CAD build for the part. Positions are in the model's coordinates, mm. Give positions to 0.01 mm unless a question says otherwise; leave off trailing zeros. Loops run counter-clockwise (first coordinate to the right, second up) from the corner with the lowest first, then second, coordinate; pieces in that order, holes last.
Item 1: Saw through at A-A on x = 0. Give the cut face in (y, z), plus the area to 3 significant figures.
Item 2: Drop flat-ended pins along their axis: P1, Ø22.5, axis at x = 171, y = -107.5, coming from the +Z side; P2, Ø1, axis at y = -57, z = 5.5, coming from the -X side; P3, Ø1.5, axis at y = 27, z = 5, coming from the -X side. Give the stop position or say it passes through.
Item 3: Probe probe 1 along X at (y, z) = (18.5, 3.75); probe 2 along Y at (x, z) = (95.5, 3.75); probe 3 along Y at (x, z) = (200, 5.5). List the from-to ranges inside material, lowest first.
Item 4: Saw through at B-B on y = 65.5. Give the cut face in (x, z), plus the area to 3 significant figures.
Item 5: Saw through at C-C on z = 5.75. Give the number of separate pieces and of enclosed holes in the cut face, plus the area to 3 significant figures.
Item 6: Saw through at D-D on x = -195.5. Give the cut face in (y, z).
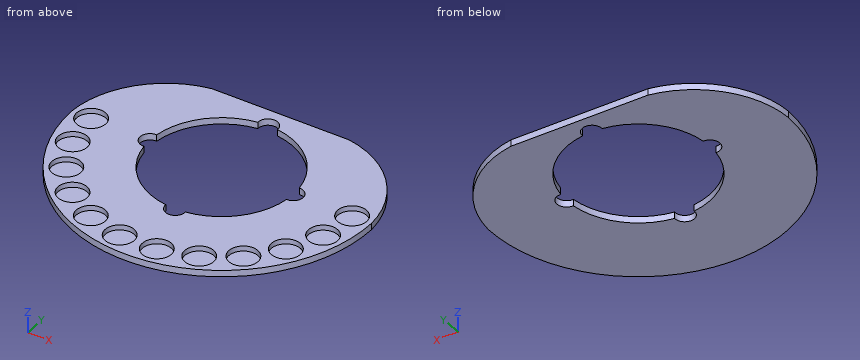
Autodesk Inventor part; units mm, degrees
ref_plane "YZ Plane" through (0, 0, 0) normal (1, 0, 0) x (0, 1, 0)
ref_plane "XZ Plane" through (0, 0, 0) normal (0, 1, 0) x (-1, 0, 0)
ref_plane "XY Plane" through (0, 0, 0) normal (0, 0, 1) x (1, 0, 0)
sketch "Sketch1" plane through (0, 0, 0) normal (0, 0, 1) x (1, 0, 0)
  line L0 (0, 0) -> (-200, 0) construction
  circle A0 centre (-200, 0) radius 17.5
  circle A1 centre (-200, 0) radius 22.5
  line L1 (0, 0) -> (-191.898595, -56.346511) construction
  circle A2 centre (-191.898595, -56.346511) radius 17.5
  circle A3 centre (-191.898595, -56.346511) radius 22.5
  line L2 (0, 0) -> (-168.250707, -108.128163) construction
  circle A4 centre (-168.250707, -108.128163) radius 17.5
  circle A5 centre (-168.250707, -108.128163) radius 22.5
  line L3 (0, 0) -> (-130.972147, -151.149915) construction
  circle A6 centre (-130.972147, -151.149915) radius 17.5
  circle A7 centre (-130.972147, -151.149915) radius 22.5
  line L4 (0, 0) -> (-83.083003, -181.926399) construction
  circle A8 centre (-83.083003, -181.926399) radius 17.5
  circle A9 centre (-83.083003, -181.926399) radius 22.5
  line L5 (0, 0) -> (-28.462968, -197.964288) construction
  circle A10 centre (-28.462968, -197.964288) radius 17.5
  circle A11 centre (-28.462968, -197.964288) radius 22.5
  line L6 (0, 0) -> (28.462968, -197.964288) construction
  circle A12 centre (28.462968, -197.964288) radius 17.5
  circle A13 centre (28.462968, -197.964288) radius 22.5
  line L7 (0, 0) -> (83.083003, -181.926399) construction
  circle A14 centre (83.083003, -181.926399) radius 17.5
  circle A15 centre (83.083003, -181.926399) radius 22.5
  line L8 (0, 0) -> (130.972147, -151.149915) construction
  circle A16 centre (130.972147, -151.149915) radius 17.5
  circle A17 centre (130.972147, -151.149915) radius 22.5
  line L9 (0, 0) -> (168.250707, -108.128163) construction
  circle A18 centre (168.250707, -108.128163) radius 17.5
  circle A19 centre (168.250707, -108.128163) radius 22.5
  line L10 (0, 0) -> (191.898595, -56.346511) construction
  circle A20 centre (191.898595, -56.346511) radius 17.5
  circle A21 centre (191.898595, -56.346511) radius 22.5
  line L11 (0, 0) -> (200, 0) construction
  circle A22 centre (200, 0) radius 17.5
  circle A23 centre (200, 0) radius 22.5
  circle A24 centre (-200, 0) radius 0 construction
  circle A25 centre (200, 0) radius 0 construction
  arc A26 (-200, 0) -> (-200, 0) centre (-200, 0) ccw
  arc A27 (200, 0) -> (200, 0) centre (200, 0) ccw
  line L12 (0, 0) -> (-200, 0) construction
  circle A28 centre (0, 0) radius 110.3
  circle A29 centre (-110, 0) radius 15.1
  arc A30 (-230, 0) -> (230, 0) centre (0, 0) ccw
  line L13 (0, 0) -> (0, 140)
  line L14 (0, 140) -> (-105, 140)
  line L15 (0, 140) -> (105, 140)
  arc A31 (230, 0) -> (105, 140) centre (80.210153, -7.937363) ccw
  arc A32 (-105, 140) -> (-230, 0) centre (-80.210153, -7.937363) ccw
  circle A33 centre (0, -110) radius 15.1
  circle A34 centre (110, 0) radius 15.1
  circle A35 centre (0, 110) radius 15.1
  point P0 (-166.666667, 74.535599)
  point P1 (-109.264, -15.082052)
  point P2 (-109.264, 15.082052)
  point P3 (15.082052, 109.264)
  point P4 (109.264, 15.082052)
  point P5 (109.264, -15.082052)
  point P6 (15.082052, -109.264)
  point P7 (-15.082052, -109.264)
  point P8 (-15.082052, 109.264)
  dimension "d1" = 35
  dimension "d2" = 45
  dimension "d5" = 180
  dimension "d35" = 200
  dimension "d36" = 220.6
  dimension "d43" = 30.2
  dimension "d48" = 230
  dimension "d49" = 140
  dimension "d53" = 105
  dimension "d54" = 150
  dimension "d55" = 150
  dimension "d56" = 210
  dimension "d58" = 110
  dimension "d61" = 360
sketch "Sketch1 outline for Extrusion1" plane through (0, 0, 0) normal (0, 0, 1) x (1, 0, 0)
  line L0 (0, 140) -> (-105, 140)
  line L1 (105, 140) -> (0, 140)
  arc A0 (-105, 140) -> (-230, 0) centre (-80.210153, -7.937363) ccw
  arc A1 (230, 0) -> (105, 140) centre (80.210153, -7.937363) ccw
  arc A2 (-230, 0) -> (230, 0) centre (0, 0) ccw
  circle A3 centre (-130.972147, -151.149915) radius 22.5
  circle A4 centre (-83.083003, -181.926399) radius 22.5
  circle A5 centre (-28.462968, -197.964288) radius 22.5
  circle A6 centre (-168.250707, -108.128163) radius 22.5
  circle A7 centre (-191.898595, -56.346511) radius 22.5
  circle A8 centre (28.462968, -197.964288) radius 22.5
  circle A9 centre (83.083003, -181.926399) radius 22.5
  circle A10 centre (130.972147, -151.149915) radius 22.5
  circle A11 centre (168.250707, -108.128163) radius 22.5
  circle A12 centre (191.898595, -56.346511) radius 22.5
  circle A13 centre (-200, 0) radius 22.5
  arc A14 (-15.082052, 109.264) -> (15.082052, 109.264) centre (0, 110) cw
  arc A15 (-109.264, 15.082052) -> (-15.082052, 109.264) centre (0, 0) cw
  arc A16 (-109.264, -15.082052) -> (-109.264, 15.082052) centre (-110, 0) cw
  arc A17 (-15.082052, -109.264) -> (-109.264, -15.082052) centre (0, 0) cw
  arc A18 (15.082052, -109.264) -> (-15.082052, -109.264) centre (0, -110) cw
  arc A19 (109.264, -15.082052) -> (15.082052, -109.264) centre (0, 0) cw
  arc A20 (109.264, 15.082052) -> (109.264, -15.082052) centre (110, 0) cw
  arc A21 (15.082052, 109.264) -> (109.264, 15.082052) centre (0, 0) cw
  circle A22 centre (200, 0) radius 22.5
extrude "Extrusion1" add sketch "Sketch1 outline for Extrusion1" along normal blind 10
sketch "Sketch1 outline for Extrusion2" plane through (0, 0, 0) normal (0, 0, 1) x (1, 0, 0)
  circle A0 centre (-200, 0) radius 22.5
  circle A1 centre (-191.898595, -56.346511) radius 22.5
  circle A2 centre (-168.250707, -108.128163) radius 22.5
  circle A3 centre (-130.972147, -151.149915) radius 22.5
  circle A4 centre (-83.083003, -181.926399) radius 22.5
  circle A5 centre (-28.462968, -197.964288) radius 22.5
  circle A6 centre (28.462968, -197.964288) radius 22.5
  circle A7 centre (83.083003, -181.926399) radius 22.5
  circle A8 centre (130.972147, -151.149915) radius 22.5
  circle A9 centre (168.250707, -108.128163) radius 22.5
  circle A10 centre (191.898595, -56.346511) radius 22.5
  circle A11 centre (200, 0) radius 22.5
extrude "Extrusion2" add sketch "Sketch1 outline for Extrusion2" along normal blind 2
properties part number "BasePlate"
Results below:
1. outline: (-230, 0) - (-125.1, 0) - (-125.1, 10) - (-230, 10) - close; (125.1, 0) - (140, 0) - (140, 10) - (125.1, 10) - close
1. area: 1,200 mm2
2. P1: stops at z = 2
2. P2: stops at x = -222.95
2. P3: stops at x = -226.26
3. probe 1: x = -227.86 to -212.81, -187.19 to -108.74, 108.74 to 187.19, 212.81 to 227.86
3. probe 2: y = -209.24 to -200.69, -163.16 to -55.19, 55.19 to 140
3. probe 3: y = -113.58 to -77.34, -35.36 to -22.5, 22.5 to 82.34
4. outline: (-211, 0) - (-88.75, 0) - (-88.75, 10) - (-211, 10) - close; (88.75, 0) - (211, 0) - (211, 10) - (88.75, 10) - close
4. area: 2,450 mm2
5. separate pieces: 1
5. enclosed holes: 13
5. area: 79,700 mm2
6. outline: (-121.16, 0) - (88.02, 0) - (88.02, 10) - (22.05, 10) - (22.05, 2) - (-22.05, 2) - (-22.05, 10) - (-34.14, 10) - (-34.14, 2) - (-78.56, 2) - (-78.56, 10) - (-121.16, 10) - close
